from build123d import *

# Parameters (mm, degrees)
SKETCH_1_R            = 3
EXTRUDE_251_DEPTH     = 2.5
CHAMFER_1_SIZE        = 1.5
CUT_EXTRUDE_459_DEPTH = 1.3
SKETCH_3_R            = 1.5
EXTRUDE_571_DEPTH     = 18


with BuildPart() as part:
    # 草图1 → Extrude 251 (new body)
    with BuildSketch(Plane(origin=(0, 0, 0), x_dir=(1, 0, 0), z_dir=(0, 1, 0))):
        Circle(SKETCH_1_R)
    extrude(amount=EXTRUDE_251_DEPTH)

    # 倒角1
    chamfer_1_edges = [part.edges().sort_by_distance(p)[0] for p in [
        (-3, 0, 0),
    ]]
    chamfer(chamfer_1_edges, length=CHAMFER_1_SIZE)

    # 草图2 → Cut-Extrude 459 (cut)
    with BuildSketch(Plane(origin=(0, 2.5, 0), x_dir=(1, 0, 0), z_dir=(0, 1, 0))):
        Polygon((1.443375673, 0), (0.721687836, 1.25), (-0.721687836, 1.25), (-1.443375673, 0), (-0.721687836, -1.25), (0.721687836, -1.25), align=None)
    extrude(amount=-CUT_EXTRUDE_459_DEPTH, mode=Mode.SUBTRACT)

    # 草图3 → Extrude 571 (add)
    with BuildSketch(Plane.XZ):
        Circle(SKETCH_3_R)
    extrude(amount=EXTRUDE_571_DEPTH)


solid = part.part
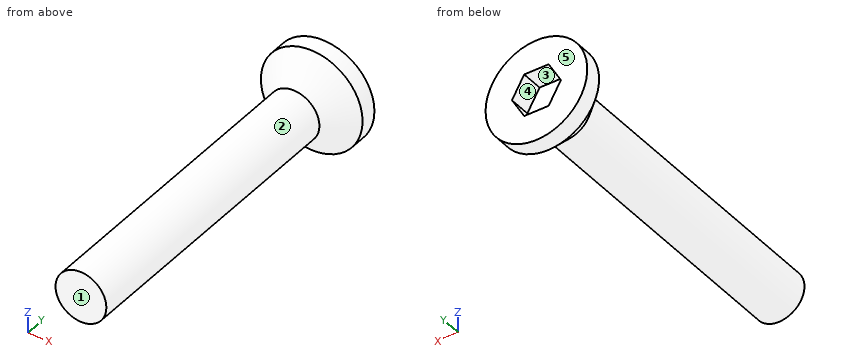
Model file for the job. Use its own axes, mm. Face numbers are marked on the shaded views. A direction names the side the tool comes from. Give positions to 0.01 mm unless a question says otherwise; leave off trailing zeros. Order: outer loops, then holes, each group sorted by start corner. A loop starts at its lowest first (then second) coordinate and runs counter-clockwise, first axis right, second up. Notation, with made-up numbers: M 75,47 L 120,47 A19 ccw 120,63 Z; hole C 4,76 d3. An arc over 180 degrees is marked long. Put each result on its own line as item: value. Start each with the question number.
(1) Band-saw the part on A-A on x = 0. Give the cut face in (y, z).
(2) Drill centre lines: L1, parallel to Y at x = 1, z = 0.2; L2, parallel to Z at x = 0.1, y = -11.5; L3, parallel to Z at x = -0.75, y = -4.75. Where is each one in solid material? Low to high. Write a range as [from, to].
(3) Tool access for the marked faces 4 and 5: list every direction of +Z, -Z, +X, -X, +Y, -Y with a clear straight run to the whole face (end or side of a thin tool).
(4) Band-saw the part on B-B on y = -14.75. Give the cut face in (x, z).
(5) Pull direction Z, two halves, no side cores. Call the marked faces 1, 2 and 3: released by +Z, released by -Z, zero draft, split by the parting line, or undercut.
(6) Pin check, flat tips, straight feed: pin 1 Ø1.5 at (y, z) = (-13, -2) entering from +X; pin 2 Ø1.5 at (x, y) = (0.5, -11.5) entering from +Z; pin 3 Ø1.5 at (y, z) = (-8.5, 0.5) entering from +X. Stop position of each tip, or through.
Results below:
1. outline: M -18,-1.5 L 0,-1.5 L 1.5,-3 L 2.5,-3 L 2.5,-1.25 L 1.2,-1.25 L 1.2,1.25 L 2.5,1.25 L 2.5,3 L 1.5,3 L 0,1.5 L -18,1.5 Z
2. L1: y = [-18, 1.2]
2. L2: z = [-1.5, 1.5]
2. L3: z = [-1.3, 1.3]
3. face 4: +Y
3. face 5: +Z, -Z, +X, -X, +Y
4. outline: C 0,0 d3
5. face 1: zero draft
5. face 2: split by the parting line
5. face 3: undercut
6. pin 1: stops at x = 0.83
6. pin 2: stops at z = 1.5
6. pin 3: stops at x = 1.5
